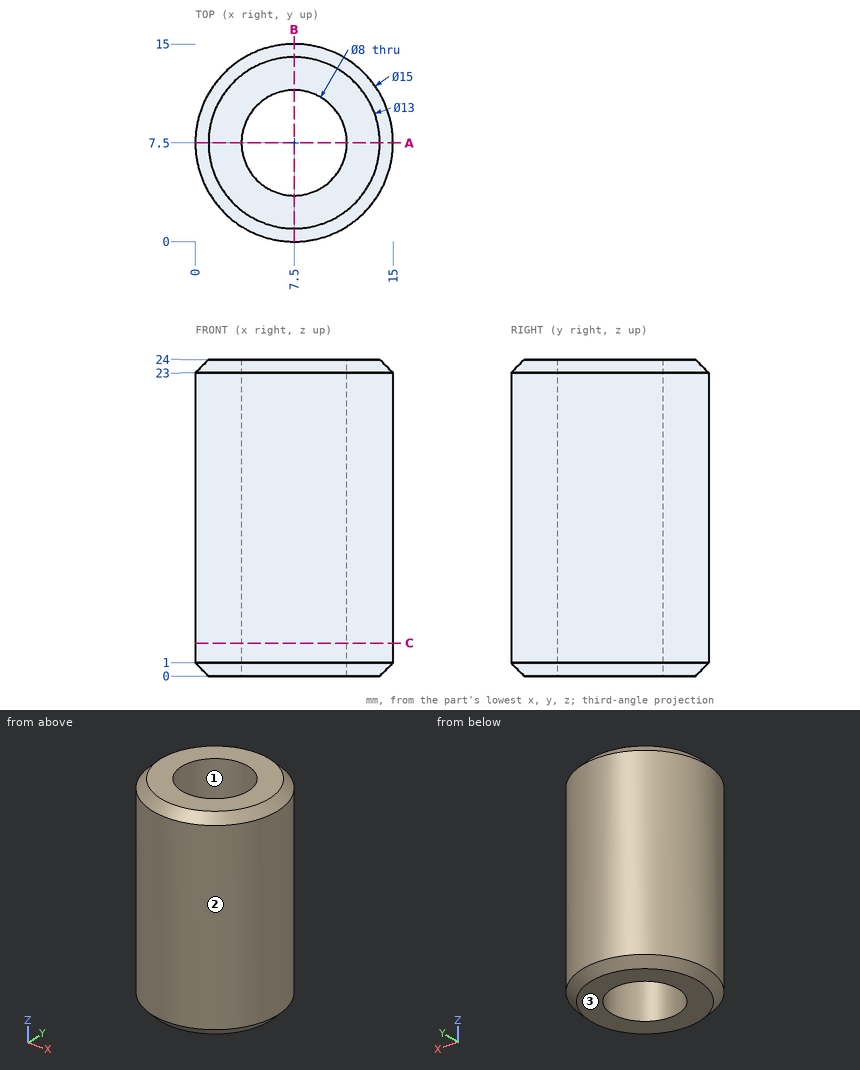
Drawing for the job (mm, zero at the part's lowest x, y, z). Give positions to 0.01 mm unless a question says otherwise; leave off trailing zeros. Loops run counter-clockwise (first coordinate to the right, second up) from the corner with the lowest first, then second, coordinate; pieces in that order, holes last.
Item 1: Mould opens along Y. For the marked faces 1, 2 and 3 say: +Y half, -Y half, draft (parallel to the pull), parting line (faces both ways), or undercut.
Check values:
face 1: undercut
face 2: parting line
face 3: draft
Item 2: Drill centre lines: line 1 along Y through (x, z) = (7.5, 7.25); line 2 along Y through (x, z) = (5.5, 21); line 3 along Y through (x, z) = (13, 8). Where is each one in solid material? Low to high.
Check values:
line 1: y = 0 to 3.5, 11.5 to 15
line 2: y = 0.27 to 4.04, 10.96 to 14.73
line 3: y = 2.4 to 12.6
Item 3: Slice it at C-C (z = 2.5). Write the cut outline in (x, y).
Check values:
outline: circle Ø15 at (7.5, 7.5); hole circle Ø8 at (7.5, 7.5)
Item 4: Drop flat-ended pins along their axis: P1, Ø3, axis at y = 4, z = 19, coming from the +X side; P2, Ø4, axis at y = 13, z = 9.5, coming from the -X side. Give the stop position or say it passes through.
Check values:
P1: stops at x = 14.73
P2: stops at x = 0.87
Item 5: Slice it at A-A (y = 7.5). Write the cut outline in (x, z), plus the area to 3 significant figures.
Check values:
outline: (0, 1) - (1, 0) - (3.5, 0) - (3.5, 24) - (1, 24) - (0, 23) - close; (11.5, 0) - (14, 0) - (15, 1) - (15, 23) - (14, 24) - (11.5, 24) - close
area: 166 mm2
